Autodesk Fusion 360 part; units mm, degrees
sketch "Sketch2" plane through (0, 0, 0) normal (0, 0, 1) x (1, 0, 0)
  line L0 (-0.6794, 183.904) -> (9.8206, 183.904)
  line L1 (9.8206, 183.904) -> (9.8206, 182.304)
  line L2 (9.8206, 182.304) -> (-0.6794, 182.304)
  line L3 (-0.6794, 182.304) -> (-0.6794, 183.904)
  line L4 (12.8206, 179.304) -> (-3.6794, 179.304)
  line L5 (-3.6794, 179.304) -> (-3.6794, 186.904)
  line L6 (-3.6794, 186.904) -> (12.8206, 186.904)
  line L7 (12.8206, 186.904) -> (12.8206, 179.304)
  line L8 (-3.6794, 182.304) -> (12.8206, 182.304)
  line L9 (12.8206, 182.304) -> (12.8206, 152.304)
  line L10 (12.8206, 152.304) -> (-3.6794, 152.304)
  line L11 (-3.6794, 152.304) -> (-3.6794, 182.304)
  line L12 (9.8206, 186.904) -> (9.8206, 152.304)
  dimension "d63" = 10.5
  dimension "d64" = 1.6
  dimension "d66" = 30
extrude "Extrude12" add sketch "Sketch2" along normal blind 10 contours L0 L3 L5 L6 L8 L12 | L2 L4 L5 L8 L11 L12 | L4 L10 L11 L12
fillet "Fillet1" radius 1.5 3 edges at (9.8206, 183.904, 5) (9.8206, 186.904, 5) (9.8206, 182.304, 5)
fillet "Fillet2" radius 3 1 edges at (-3.6794, 186.904, 5)
chamfer "Chamfer2" distance 0.5 angle 45 18 edges at (-3.6794, 168.104, 0) (-2.8008, 186.0253, 0) (3.8206, 186.904, 0) (9.8206, 185.404, 0) (3.8206, 183.904, 0) (-0.6794, 183.104, 0) (3.8206, 182.304, 0) (9.3812, 181.8646, 0) (9.8206, 166.554, 0) (-3.6794, 168.104, 10) (-2.8008, 186.0253, 10) (3.8206, 186.904, 10) (9.8206, 185.404, 10) (3.8206, 183.904, 10) (3.8206, 182.304, 10) (9.3812, 181.8646, 10) (9.8206, 166.554, 10) (-0.6794, 183.104, 10)
sketch "Sketch3" plane through (0, 183.904, 0) normal (0, -1, 0) x (1, 0, 0)
  line L0 (8.3206, 9.5) -> (-0.6794, 9.5)
  line L1 (-0.6794, 9.5) -> (-0.6794, 0.5)
  line L2 (-0.6794, 0.5) -> (8.3206, 0.5)
  line L3 (8.3206, 0.5) -> (8.3206, 9.5)
  line L4 (-0.6794, 9.5) -> (8.3206, 0.5) construction
  line L5 (-0.6794, 0.5) -> (8.3206, 9.5) construction
  line L6 (8.3206, 5) -> (3.8206, 5) construction
  circle A0 centre (6.3206, 5) radius 2
  dimension "d75" = 4
extrude "Extrude13" add sketch "Sketch3" along normal blind 0.5 contours A0
chamfer "Chamfer3" distance 0.5 angle 45 1 edges at (4.4559, 183.404, 4.2768)
equation "d63 = slot_depth"
equation "d64 = pcb_thickness"
equation "d66 = leg_height"
equation "d67 = leg_thickness"
equation "leg_height = 30 mm"
equation "pcb_thickness = 1.6 mm"
equation "wall_thickness = 3 mm"
equation "slot_depth = 10.5 mm"
equation "leg_thickness = 10 mm"
For this review, take the finished solid that the model builds, in its own axes (mm). A direction names the side the tool comes from. Round coordinates to 2 decimals unless told otherwise and drop trailing zeros. Write each loop counter-clockwise with the first axis right and the second up, starting at its lowest first coordinate (ties: lowest second). Pieces come first, ordered by that corner, then holes. Notation, with made-up numbers: (82.25, 11.5) - (87.25, 11.5) arc R30 ccw to (87.25, 45.5) - close; hole circle Ø1 at (-35, 70.25). An arc over 180 degrees is marked (long way). Answer as CSV lines item,"result". Start each with the question number.
(1) Machinability: for faces 4 (the cylindrical face through (9.393, 186.453, 5.063)), 5 (the flat face through (4, 183.904, 5)), 6 (the flat face through (4, 182.304, 5)), 7 (the conical face through (9.18, 181.64, 0.2)), 8 (the conical face through (9.18, 184.57, 9.8)), which of the approach directions +Z, -Z, +X, -X, +Y, -Y give a long, thin tool a straight path to every point of the face, cutting with its end or side? Answer none if there is none.
(2) Add section A-A, the plane x = 3. State the section outline as (y, z) points, plus the area to 3 significant figures.
(3) For line 1 (Y direction, x = 0.5, z = 3.5); line 2 (Y direction, x = 6.5, z = 5.75); line 3 (Y direction, x = -3, z = 2.75), list the stretches that pass through material, from the lowest coordinate up.
(4) Add section C-C, the plane y = 183. State the section outline as (x, z) points, plus the area to 3 significant figures.
(5) Mouldability with a two-part tool opening along Y and no side actions: class faces 1 (the conical face through (-2.53, 185.79, 0.14)), 2 (the conical face through (9.16, 184.55, 0.2)), 3 (the flat face through (9.821, 167, 5)) as +Y half, -Y half, draft (parallel to the pull), parting line (faces both ways), or undercut.
From the geometry:
1,face 4,"+Z, -Z, +X, +Y"
1,face 5,"none"
1,face 6,"+Z, -Z, +X"
1,face 7,"-Z, +X"
1,face 8,"+Z, +X"
2,outline,"(152.3, 0) - (181.8, 0) - (182.3, 0.5) - (182.3, 9.5) - (181.8, 10) - (152.3, 10) - close; (183.9, 0.5) - (184.4, 0) - (186.4, 0) - (186.9, 0.5) - (186.9, 9.5) - (186.4, 10) - (184.4, 10) - (183.9, 9.5) - close"
2,area,"329 mm²"
3,line 1,"y = 152.3 to 182.3, 183.9 to 186.9"
3,line 2,"y = 152.3 to 182.3, 183.4 to 186.9"
3,line 3,"y = 152.3 to 185.81"
4,outline,"(-3.68, 0.5) - (-3.18, 0) - (-1.18, 0) - (-0.68, 0.5) - (-0.68, 9.5) - (-1.18, 10) - (-3.18, 10) - (-3.68, 9.5) - close"
4,area,"29.5 mm²"
5,face 1,"+Y half"
5,face 2,"undercut"
5,face 3,"draft"
